Read the model definition and answer for the solid it produces. Units are mm, in the model's axes. A direction names the side the tool comes from. Coordinates: 2 decimals unless noted, no trailing zeros. Loops run counter-clockwise (first coordinate to the right, second up) from the corner with the lowest first, then second, coordinate; pieces in that order, holes last. Notation, with made-up numbers: (2.25, 81) -> (13.25, 81) arc R23 ccw to (13.25, 89) -> close; hole circle Ø2 at (-38, 46). An arc over 180 degrees is marked (long way). Answer as a JSON object with one key per item and string values. Group by question number.
1) Section D-D, the plane z = 2.25 is taken. Give the vertices of the cut face in (x, y).
2) Determine the mould class of faces 1 (the face through (-21.43, 0.03, 5.99)), 2 (the face through (15, 15, 7)), 3 (the face through (-23.977, 1.055, 2.465)) for opening direction X: released by +X, released by -X, zero draft, split by the parting line, or undercut.
3) Section A-A, the plane x = 0 is taken. Give the vertices of the cut face in (y, z) (3 decimals).
4) Consider probe 1 along Y at (x, z) = (0, 1.55); probe 2 along X at (y, z) = (12, 5.25); probe 3 along Y at (x, z) = (-6.5, 5.5). Determine where each line is inside the solid, lowest interval first. Write a range as [from, to].
5) Which of the six approach directions +Z, -Z, +X, -X, +Y, -Y give full straight-line access (tool end or side, diameter ignored) to faces 4 (the face through (8, -8, 7)), 5 (the face through (4.57, 11.03, 5.99)), 6 (the face through (10.158, 10.047, 5.986))?
6) Section C-C, the plane x = 20.73 is taken. Give the vertices of the cut face in (y, z).
7) Flat-ended cylindrical pins translate along their axes: P1, Ø2, axis at y = -1.5, z = 1, coming from the -X side; P2, Ø1.5, axis at y = 11, z = 1, coming from the +X side; P3, Ø1, axis at x = -17.5, z = 3.5, coming from the -Y side; P4, Ø10.5, axis at x = 0, y = 0, coming from the -Z side. Find the tip coordinate at first contact, or state that the pin passes through.
from build123d import *

# Parameters (mm, degrees)
SKETCH1_R          = 24
EXTRUDE1_DEPTH     = 5
SKETCH5_R          = 6.5
CUT_EXTRUDE3_DEPTH = 10
SKETCH4_R          = 0.7
EXTRUDE2_DEPTH     = 2


with BuildPart() as part:
    # Sketch1 → Extrude1 (new body)
    with BuildSketch(Plane.XY):
        Circle(SKETCH1_R)
    extrude(amount=EXTRUDE1_DEPTH)

    # Sketch5 → Cut-Extrude3 (cut)
    with BuildSketch(Plane(origin=(0, 0, 0), x_dir=(-1, 0, 0), z_dir=(0, 0, -1))):
        Circle(SKETCH5_R)
    extrude(amount=-CUT_EXTRUDE3_DEPTH, mode=Mode.SUBTRACT)

    # Sketch4 → Extrude2 (add)
    with BuildSketch(Plane.XY.offset(5)):
        with Locations((0, 20.73)):
            Circle(SKETCH4_R)
        with Locations((0, -20.73)):
            Circle(SKETCH4_R)
        with Locations((20.73, 0)):
            Circle(SKETCH4_R)
        with Locations((-20.73, 0)):
            Circle(SKETCH4_R)
        with Locations((-14.658, 14.658)):
            Circle(SKETCH4_R)
        with Locations((14.658, 14.658)):
            Circle(SKETCH4_R)
        with Locations((14.658, -14.658)):
            Circle(SKETCH4_R)
        with Locations((-14.658, -14.658)):
            Circle(SKETCH4_R)
        with Locations((19.152, 7.933)):
            Circle(SKETCH4_R)
        with Locations((7.933, 19.152)):
            Circle(SKETCH4_R)
        with Locations((19.152, -7.933)):
            Circle(SKETCH4_R)
        with Locations((7.933, -19.152)):
            Circle(SKETCH4_R)
        with Locations((-7.933, 19.152)):
            Circle(SKETCH4_R)
        with Locations((-19.152, 7.933)):
            Circle(SKETCH4_R)
        with Locations((-19.152, -7.933)):
            Circle(SKETCH4_R)
        with Locations((-7.933, -19.152)):
            Circle(SKETCH4_R)
        with Locations((0, 17.555)):
            Circle(SKETCH4_R)
        with Locations((17.555, 0)):
            Circle(SKETCH4_R)
        with Locations((0, -17.555)):
            Circle(SKETCH4_R)
        with Locations((-17.555, 0)):
            Circle(SKETCH4_R)
        with Locations((-12.413, 12.413)):
            Circle(SKETCH4_R)
        with Locations((12.413, 12.413)):
            Circle(SKETCH4_R)
        with Locations((12.413, -12.413)):
            Circle(SKETCH4_R)
        with Locations((-12.413, -12.413)):
            Circle(SKETCH4_R)
        with Locations((-16.218, 6.718)):
            Circle(SKETCH4_R)
        with Locations((16.218, 6.718)):
            Circle(SKETCH4_R)
        with Locations((16.218, -6.718)):
            Circle(SKETCH4_R)
        with Locations((-16.218, -6.718)):
            Circle(SKETCH4_R)
        with Locations((6.718, 16.218)):
            Circle(SKETCH4_R)
        with Locations((6.718, -16.218)):
            Circle(SKETCH4_R)
        with Locations((-6.718, -16.218)):
            Circle(SKETCH4_R)
        with Locations((-6.718, 16.218)):
            Circle(SKETCH4_R)
        with BuildLine():
            Line((3.645052576, -8.799955495), (5.467578865, -13.199933243))
            ThreePointArc((5.467578865, -13.199933243), (10.102788136, -10.102788136), (13.199933243, -5.467578865))
            Line((13.199933243, -5.467578865), (8.799955495, -3.645052576))
            ThreePointArc((8.799955495, -3.645052576), (6.735192091, -6.735192091), (3.645052576, -8.799955495))
        make_face()
        with BuildLine():
            Line((8.799955495, 3.645052576), (13.199933243, 5.467578865))
            ThreePointArc((13.199933243, 5.467578865), (10.102788136, 10.102788136), (5.467578865, 13.199933243))
            Line((5.467578865, 13.199933243), (3.645052576, 8.799955495))
            ThreePointArc((3.645052576, 8.799955495), (6.735192091, 6.735192091), (8.799955495, 3.645052576))
        make_face()
        with BuildLine():
            Line((-3.645052576, 8.799955495), (-5.467578865, 13.199933243))
            ThreePointArc((-5.467578865, 13.199933243), (-10.102788136, 10.102788136), (-13.199933243, 5.467578865))
            Line((-13.199933243, 5.467578865), (-8.799955495, 3.645052576))
            ThreePointArc((-8.799955495, 3.645052576), (-6.735192091, 6.735192091), (-3.645052576, 8.799955495))
        make_face()
        with BuildLine():
            Line((-8.799955495, -3.645052576), (-13.199933243, -5.467578865))
            ThreePointArc((-13.199933243, -5.467578865), (-10.102788136, -10.102788136), (-5.467578865, -13.199933243))
            Line((-5.467578865, -13.199933243), (-3.645052576, -8.799955495))
            ThreePointArc((-3.645052576, -8.799955495), (-6.735192091, -6.735192091), (-8.799955495, -3.645052576))
        make_face()
    extrude(amount=EXTRUDE2_DEPTH)


solid = part.part
Determined:
{
 "1": {"outline": "circle Ø48 at (0, 0); hole circle Ø13 at (0, 0)"},
 "2": {"face 1": "undercut", "face 2": "zero draft", "face 3": "split by the parting line"},
 "3": {"outline": "(-24, 0) -> (-6.5, 0) -> (-6.5, 5) -> (-16.855, 5) -> (-16.855, 7) -> (-18.255, 7) -> (-18.255, 5) -> (-20.03, 5) -> (-20.03, 7) -> (-21.43, 7) -> (-21.43, 5) -> (-24, 5) -> close; (6.5, 0) -> (24, 0) -> (24, 5) -> (21.43, 5) -> (21.43, 7) -> (20.03, 7) -> (20.03, 5) -> (18.255, 5) -> (18.255, 7) -> (16.855, 7) -> (16.855, 5) -> (6.5, 5) -> close"},
 "4": {"probe 1": "[-24, -6.5], [6.5, 24]", "probe 2": "[-12.98, -11.85], [-7.75, -4.97], [4.97, 7.75], [11.85, 12.98]", "probe 3": "[-16.88, -15.55], [-12.72, -6.96], [6.96, 12.72], [15.55, 16.88]"},
 "5": {"face 4": "+Z, +X, -X, +Y, -Y", "face 5": "+Z, +Y", "face 6": "+Z"},
 "6": {"outline": "(-12.09, 0) -> (12.09, 0) -> (12.09, 5) -> (0.7, 5) -> (0.7, 7) -> (-0.7, 7) -> (-0.7, 5) -> (-12.09, 5) -> close"},
 "7": {"P1": "x = -23.99", "P2": "x = 21.7", "P3": "y = -16.94", "P4": "through"}
}
